Verification items for the finished model (mm, model axes). A direction names the side the tool comes from. Round coordinates to 2 decimals unless told otherwise and drop trailing zeros. Write each loop counter-clockwise with the first axis right and the second up, starting at its lowest first coordinate (ties: lowest second). Pieces come first, ordered by that corner, then holes. Notation, with made-up numbers: M 25,78.25 L 48,78.25 A19 cw 48,88.25 Z; hole C 59,-36.5 d8. An arc over 180 degrees is marked long. Answer in a Markdown table with one row per item. Add a question column.
1. Sectioned sample at D-D on x = 0. Record the cut outline in (y, z), plus the area to 3 significant figures.
2. Set-up check for faces 1 (the flat face through (0.75, 15, 6)), 2 (the cylindrical face through (-3.919, 14.024, 7.283)), 3 (the flat face through (1.2, 22, -3.4)), 4 (the flat face through (-0.75, 15, -18)): record each of +Z, -Z, +X, -X, +Y, -Y from which the full face is reachable in a straight line by a thin tool's end or side.
3. Material ranges on probe 1 along X at (y, z) = (15.5, 0); probe 2 along X at (y, z) = (17.25, 7.5); probe 3 along Y at (x, z) = (-3, 7.5), recorded low to high.
4. Sectioned sample at B-B on z = -3. Record the cut outline in (x, y).
5. Sectioned sample at A-A on y = 15. Record the cut outline in (x, z), plus the area to 3 significant figures.
6. Draft check along X on faces 5 (the flat face through (-4, 15, 10)), 6 (the flat face through (-7, 15, -6)), 7 (the flat face through (-0.75, 15, 6)). Enter one of: pulls with the +X half, pulls with the -X half, needs draft (parallel to the pull), parting line crosses it, or undercut.
7. Go/stop test with a flat-tipped pin: pin 1 Ø1.2 at (y, z) = (15, 7.5) entering from +X. Record where the tip stops, or that it passes through.
8. Sectioned sample at C-C on z = 7.5. Record the cut outline in (x, y), plus the area to 3 significant figures.
```python
from build123d import *

# Parameters (mm, degrees)
SKETCH1_W           = 14
SKETCH1_H           = 32
SKETCH1_R           = 3.4
SKETCH1_R_2         = 4
BOSS_EXTRUDE1_DEPTH = 30
SKETCH2_R           = 5
CUT_EXTRUDE1_DEPTH  = 8
SKETCH3_W           = 1.5
SKETCH3_H           = 20
CUT_EXTRUDE2_DEPTH  = 38.854986461
SKETCH4_R           = 1
CUT_EXTRUDE3_DEPTH  = 40.749213829


with BuildPart() as part:
    # Sketch1 → Boss-Extrude1 (new body)
    with BuildSketch(Plane(origin=(0, 0, 0), x_dir=(1, 0, 0), z_dir=(0, 1, 0))):
        with Locations((0, 6)):
            Rectangle(SKETCH1_W, SKETCH1_H)
        with Locations(Location((0, 0, 0), (0, 0, 270))):
            Circle(SKETCH1_R, mode=Mode.SUBTRACT)
        with Locations(Location((0, 12, 0), (0, 0, 270))):
            Circle(SKETCH1_R_2, mode=Mode.SUBTRACT)
    extrude(amount=BOSS_EXTRUDE1_DEPTH)

    # Sketch2 → Cut-Extrude1 (cut)
    with BuildSketch(Plane(origin=(0, 30, 0), x_dir=(1, 0, 0), z_dir=(0, 1, 0))):
        with Locations(Location((0, 0, 0), (0, 0, 270))):
            Circle(SKETCH2_R)
    extrude(amount=-CUT_EXTRUDE1_DEPTH, mode=Mode.SUBTRACT)

    # Sketch3 → Cut-Extrude2 (cut, through all)
    with BuildSketch(Plane.XZ):
        with Locations((0, 10)):
            Rectangle(SKETCH3_W, SKETCH3_H)
        with Locations((0, -22)):
            Rectangle(SKETCH3_W, SKETCH3_H)
    extrude(amount=-CUT_EXTRUDE2_DEPTH, mode=Mode.SUBTRACT)

    # Sketch4 → Cut-Extrude3 (cut, through all)
    with BuildSketch(Plane.ZY.offset(7)):
        with Locations((7.5, 15)):
            Circle(SKETCH4_R)
        with Locations((-19.5, 15)):
            Circle(SKETCH4_R)
    extrude(amount=-CUT_EXTRUDE3_DEPTH, mode=Mode.SUBTRACT)


solid = part.part
```
Geometry check:
| question | item | result |
|---|---|---|
| 1 | outline | M 0,-8 L 30,-8 L 30,-5 L 22,-5 L 22,-3.4 L 0,-3.4 Z |
| 1 | area | 125 mm2 |
| 2 | face 1 | +Z, +Y, -Y |
| 2 | face 2 | +X, -X |
| 2 | face 3 | +Y |
| 2 | face 4 | -Z, +Y, -Y |
| 3 | probe 1 | x = -7 to -3.4, 3.4 to 7 |
| 3 | probe 2 | x = -7 to -0.75, 0.75 to 7 |
| 3 | probe 3 | y = 0 to 14, 16 to 30 |
| 4 | outline | M -7,0 L -1.6,0 L -1.6,22 L -4,22 L -4,30 L -7,30 Z; M 1.6,0 L 7,0 L 7,30 L 4,30 L 4,22 L 1.6,22 Z |
| 5 | outline | M -7,-22 L -0.75,-22 L -0.75,-20.5 L -7,-20.5 Z; M -7,-18.5 L -0.75,-18.5 L -0.75,-15.93 A4 cw long 0.75,-15.93 L 0.75,-18.5 L 7,-18.5 L 7,6.5 L 0.75,6.5 L 0.75,3.32 A3.4 cw long -0.75,3.32 L -0.75,6.5 L -7,6.5 Z; M -7,8.5 L -0.75,8.5 L -0.75,10 L -7,10 Z; M 0.75,-22 L 7,-22 L 7,-20.5 L 0.75,-20.5 Z; M 0.75,8.5 L 7,8.5 L 7,10 L 0.75,10 Z |
| 5 | area | 292 mm2 |
| 6 | face 5 | needs draft |
| 6 | face 6 | pulls with the -X half |
| 6 | face 7 | undercut |
| 7 | pin 1 | passes through |
| 8 | outline | M -7,0 L -0.75,0 L -0.75,14 L -7,14 Z; M -7,16 L -0.75,16 L -0.75,30 L -7,30 Z; M 0.75,0 L 7,0 L 7,14 L 0.75,14 Z; M 0.75,16 L 7,16 L 7,30 L 0.75,30 Z |
| 8 | area | 350 mm2 |
